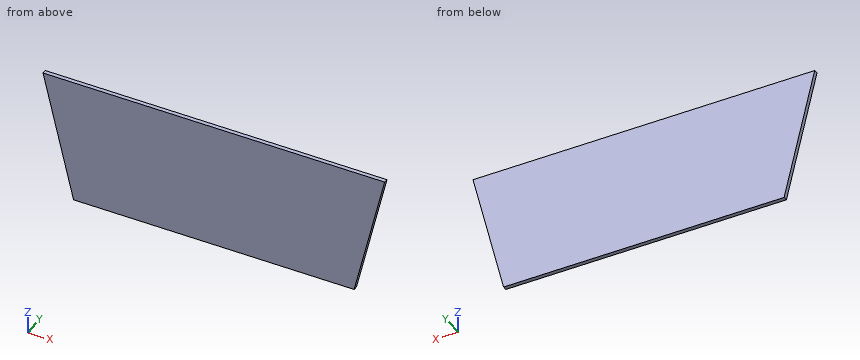
from build123d import *

# Parameters (mm, degrees)
F0_W     = 540
F0_H     = 390
F1_DEPTH = 10
F3_DEPTH = 10
F4_DEPTH = 10.001
F5_DEPTH = 10


with BuildPart() as f1:
    # F0 (on Front) → F1 (new body)
    with BuildSketch(Plane.XZ):
        Polygon((-575.5810141563, 243.9473703504), (-465.5810141563, -206.0526296496), (133.660423523, -206.0526296496), (243.660423523, 243.9473703504), (133.660423523, 243.9473703504), (-465.5810141563, 243.9473703504), align=None)
        with Locations((-166.339576477, 18.9473703504)):
            Rectangle(F0_W, F0_H, mode=Mode.SUBTRACT)
        Polygon((-495.5810141563, 43.0153865893), (-537.3643879646, 213.9473703504), (-495.5810141563, 213.9473703504), align=None, mode=Mode.SUBTRACT)
        Polygon((163.660423523, 213.9473703504), (205.4437973313, 213.9473703504), (163.660423523, 43.0153865893), align=None, mode=Mode.SUBTRACT)
    extrude(amount=F1_DEPTH)

    # F2 (on face) → F3 (join)
    with BuildSketch(Plane.XZ.offset(10)):
        Polygon((-436.339576477, 213.9473703504), (-436.339576477, -56.0526296496), (-237.4058812857, -56.0526296496), (103.660423523, -56.0526296496), (103.660423523, 213.9473703504), align=None)
        Polygon((-237.4058812857, 243.9473703504), (-575.5810141563, 243.9473703504), (-502.247680823, -56.0526296496), (-436.339576477, -56.0526296496), (-436.339576477, 213.9473703504), (103.660423523, 213.9473703504), (103.660423523, -56.0526296496), (170.3270901897, -56.0526296496), (243.660423523, 243.9473703504), align=None)
        Polygon((-495.5810141563, 213.9473703504), (-495.5810141563, 43.0153865893), (-537.3643879646, 213.9473703504), align=None, mode=Mode.SUBTRACT)
        Polygon((163.660423523, 43.0153865893), (163.660423523, 213.9473703504), (205.4437973313, 213.9473703504), align=None, mode=Mode.SUBTRACT)
        Polygon((-537.3643879646, 213.9473703504), (-495.5810141563, 43.0153865893), (-495.5810141563, 213.9473703504), align=None)
        Polygon((205.4437973313, 213.9473703504), (163.660423523, 213.9473703504), (163.660423523, 43.0153865893), align=None)
    extrude(amount=F3_DEPTH)

    # F4 (cut, through all): a face of the model
    f4_faces = [f1.faces().sort_by_distance(p)[0] for p in [
        (-469.29362865, -10, -62.9436152294),
    ]]
    extrude(f4_faces, amount=-F4_DEPTH, mode=Mode.SUBTRACT)

    # F0 (on Front) → F5 (cut)
    with BuildSketch(Plane.XZ):
        Polygon((-575.5810141563, 243.9473703504), (-465.5810141563, -206.0526296496), (133.660423523, -206.0526296496), (243.660423523, 243.9473703504), (133.660423523, 243.9473703504), (-465.5810141563, 243.9473703504), align=None)
        with Locations((-166.339576477, 18.9473703504)):
            Rectangle(F0_W, F0_H, mode=Mode.SUBTRACT)
        Polygon((-495.5810141563, 43.0153865893), (-537.3643879646, 213.9473703504), (-495.5810141563, 213.9473703504), align=None, mode=Mode.SUBTRACT)
        Polygon((163.660423523, 213.9473703504), (205.4437973313, 213.9473703504), (163.660423523, 43.0153865893), align=None, mode=Mode.SUBTRACT)
    extrude(amount=F5_DEPTH, mode=Mode.SUBTRACT)


solid = f1.part
Geometry check sheet. Reference: the model listing, model coordinates, mm. Coordinates: 2 decimals unless noted, no trailing zeros. Order: outer loops, then holes, each group sorted by start corner. A loop starts at its lowest first (then second) coordinate and runs counter-clockwise, first axis right, second up. Notation, with made-up numbers: M -18.5,31.5 L -5.5,31.5 A14 cw -5.5,44.5 Z; hole C 46,40 d4. An arc over 180 degrees is marked long. Use CSV: the item, a comma, the result in double quotes.
Item 1: Cross-section at B-B on z = 144. Record the cut outline in (x, y), then the cut area to 3 significant figures.
Returned:
outline,"M -551.15,-20 L 219.23,-20 L 219.23,-10 L -551.15,-10 Z"
area,"7,700 mm2"
Item 2: Cross-section at A-A on y = -12. Record the cut outline in (x, z), then the cut area to 3 significant figures.
Returned:
outline,"M -575.58,243.95 L -502.25,-56.05 L 170.33,-56.05 L 243.66,243.95 Z"
area,"224,000 mm2"
Item 3: Gauge pin test, flat ends, axial feed: pin 1 Ø3 at (y, z) = (-17.5, 149) entering from +X; pin 2 Ø1.5 at (y, z) = (-16, 136.5) entering from +X; pin 3 Ø5 at (y, z) = (-18.5, -2) entering from -X. Record the tip position at first contact, or that the pin passes through.
Returned:
pin 1,"stops at x = 220.82"
pin 2,"stops at x = 217.58"
pin 3,"stops at x = -516.07"
Item 4: Thickness scan on line 1 along X through (y, z) = (-18, 134.5); line 2 along X through (y, z) = (-17.75, 217). Record the ranges inside material, lowest first.
Returned:
line 1,"x = -548.83 to 216.91"
line 2,"x = -568.99 to 237.07"
